Source: CAD feature listing. Evaluate the final solid. Frame: model axes, mm. Face numbers are marked on the shaded views. A direction names the side the tool comes from. Give positions to 0.01 mm unless a question says otherwise; leave off trailing zeros. Loops run counter-clockwise (first coordinate to the right, second up) from the corner with the lowest first, then second, coordinate; pieces in that order, holes last. Notation, with made-up numbers: (76.25, 49.5) -> (81.25, 49.5) arc R16 ccw to (81.25, 79.5) -> close; hole circle Ø6 at (64, 17.5). An arc over 180 degrees is marked (long way). Return JSON: item names as keys, results as strings. Group by question number.
(1) Pin query (flat end, axial travel): pin 1 (14 mm diameter, centred on y = 20, z = 37.5, fed in from -X); pin 2 (1.5 mm diameter, centred on x = 1.5, z = -2.5, fed in from +Y); pin 3 (18 mm diameter, centred on x = 3.5, y = 54, fed in from -Z); pin 4 (12 mm diameter, centred on y = -18, z = -31.5, fed in from -X). Return the tip coordinate at first contact, or that it passes through.
(2) Draft query along Y for the marked faces 6, 7, 8 and 9. Return one class per face: released by +Y, released by -Y, zero draft, split by the parting line, or undercut.
(3) Cut plane C-C on x = -2.5. Give the number of separate pieces and of enclosed holes in the cut face, then the cut area to 3 significant figures.
(4) Access query for the marked faces 1, 2, 3, 4 and 5. Directions: +Z, -Z, +X, -X, +Y, -Y. A direction counts if a zero-diameter tool reaches every point of the face in a straight line with its end or side. Return the directions, or none.
(5) Cut plane B-B on x = -62. Return loops of the section in (y, z), then the cut area to 3 significant figures.
(6) Ray query, line 1 (Y direction, x = 5, z = 0); line 2 (Z direction, x = -11, y = 0); line 3 (X direction, y = 10, z = -6.5). Return the intervals inside material, ascending. Write a range as from..to.
(7) Cut plane A-A on y = 65. Return loops of the section in (x, z), then the cut area to 3 significant figures.
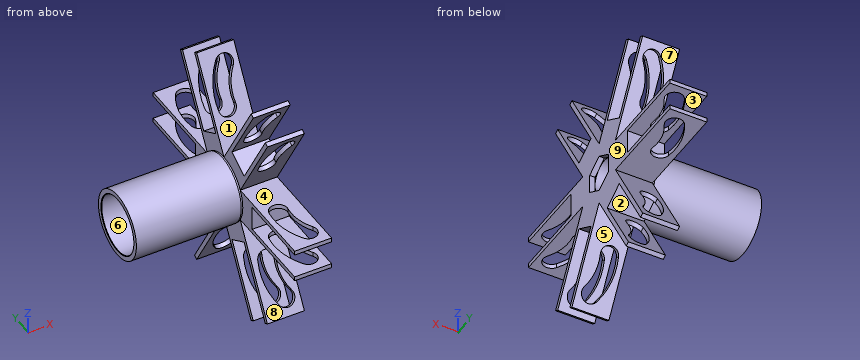
```python
from build123d import *

# Parameters (mm, degrees)
SKETCH_1_R               = 20
EXTRUDE_1_DEPTH          = 10
SKETCH_2_W               = 22.2
SKETCH_2_H               = 65
EXTRUDE_2_DEPTH          = 10
SKETCH_6_W               = 14.8
SKETCH_6_H               = 90
F_14_8MM_DEPTH           = 79.735252587
CUT_EXTRUDE_2_DEPTH      = 10
PATTERN_CIRCULAR_1_COUNT = 6
CUT_EXTRUDE_3_DEPTH      = 104.404589129
CUT_EXTRUDE_3_DEPTH_BACK = 104.404589129
SKETCH_5_R               = 10


# Read off the part's stored shape, not the designer's step: the combine step
with BuildPart() as part:
    # Sketch 1 → Extrude 1 (new, symmetric)
    with BuildSketch(Plane(origin=(0, 0, 0), x_dir=(0, 0, -1), z_dir=(1, 0, 0))):
        Circle(SKETCH_1_R)
    extrude(amount=EXTRUDE_1_DEPTH, both=True)

    # Sketch 2 → Extrude 2 (add, symmetric)
    with BuildSketch(Plane.XY):
        with Locations((2.1, 42.5)):
            Rectangle(SKETCH_2_W, SKETCH_2_H)
    extrude_2 = extrude(amount=EXTRUDE_2_DEPTH, both=True)

    # Sketch 6 → 14.8mm (cut, symmetric)
    with BuildSketch(Plane(origin=(0, 0, 0), x_dir=(0, 0, -1), z_dir=(1, 0, 0))):
        with Locations((0, 75)):
            Rectangle(SKETCH_6_W, SKETCH_6_H)
    f_14_8mm = extrude(amount=F_14_8MM_DEPTH, both=True, mode=Mode.SUBTRACT)

    # Sketch 4 → Cut-Extrude 2 (cut, symmetric)
    with BuildSketch(Plane.XY):
        with BuildLine():
            ThreePointArc((0.354791324, 67.87679305), (-4.923683601, 55.030996482), (-5.230806803, 41.146384051))
            ThreePointArc((-5.230806803, 41.146384051), (0.853615949, 36.769193197), (5.230806803, 42.853615949))
            ThreePointArc((5.230806803, 42.853615949), (5.452207774, 52.862845615), (9.257389091, 62.12320695))
            ThreePointArc((9.257389091, 62.12320695), (7.682883257, 69.451298883), (0.354791324, 67.87679305))
        make_face()
    cut_extrude_2 = extrude(amount=CUT_EXTRUDE_2_DEPTH, both=True, mode=Mode.SUBTRACT)

    # Pattern Circular 1: Extrude 2, 14.8mm, Cut-Extrude 2 ×6 about axis
    pattern_circular_1_axis = Axis((0, 0, 0), (1, 0, 0))
    add([extrude_2.rotate(pattern_circular_1_axis, i * 360 / PATTERN_CIRCULAR_1_COUNT) for i in range(1, PATTERN_CIRCULAR_1_COUNT)])
    add([f_14_8mm.rotate(pattern_circular_1_axis, i * 360 / PATTERN_CIRCULAR_1_COUNT) for i in range(1, PATTERN_CIRCULAR_1_COUNT)], mode=Mode.SUBTRACT)
    add([cut_extrude_2.rotate(pattern_circular_1_axis, i * 360 / PATTERN_CIRCULAR_1_COUNT) for i in range(1, PATTERN_CIRCULAR_1_COUNT)], mode=Mode.SUBTRACT)

    # Sketch 5 → Cut-Extrude 3 (cut, two sides: drawn at the far end of the back side and taken through both)
    with BuildSketch(Plane.ZY.offset(-CUT_EXTRUDE_3_DEPTH_BACK)):
        Circle(SKETCH_5_R)
    extrude(amount=CUT_EXTRUDE_3_DEPTH + CUT_EXTRUDE_3_DEPTH_BACK, mode=Mode.SUBTRACT)

    # Combine 3_4 outline → Combine 3_4 (revolve)
    with BuildSketch(Plane.YX):
        Polygon((6.3, -10), (6, -10.3), (6, -12.7), (6.3, -13), (17.15, -13), (17.15, -72.7), (17.45, -73), (20.15, -73), (20.15, -10), align=None)
    revolve(axis=Axis((0, 0, 0), (1, 0, 0)))


solid = part.part
```
Answers:
{
 "1": {"pin 1": "x = -9", "pin 2": "y = 30", "pin 3": "z = -60.62", "pin 4": "through"},
 "2": {"face 6": "undercut", "face 7": "released by +Y", "face 8": "released by -Y", "face 9": "zero draft"},
 "3": {"separate pieces": "13", "enclosed holes": "1", "area": "2,860 mm²"},
 "4": {"face 1": "+Z, +X, -X", "face 2": "+X, -X", "face 3": "+X, -X, +Y", "face 4": "+X, -X, -Y", "face 5": "-Z, +X, -X"},
 "5": {"outline": "circle Ø40.3 at (0, 0); hole circle Ø34.3 at (0, 0)", "area": "352 mm²"},
 "6": {"line 1": "-30..-10, 10..30", "line 2": "-20.15..-6, 6..20.15", "line 3": "-13..13.2"},
 "7": {"outline": "(-9, -10) -> (-1.33, -10) -> (-1.33, -7.4) -> (-9, -7.4) -> close; (-9, 7.4) -> (-1.33, 7.4) -> (-1.33, 10) -> (-9, 10) -> close; (10.11, -10) -> (13.2, -10) -> (13.2, -7.4) -> (10.11, -7.4) -> close; (10.11, 7.4) -> (13.2, 7.4) -> (13.2, 10) -> (10.11, 10) -> close", "area": "56.0 mm²"}
}
